from build123d import *

# Parameters (mm, degrees)
F0_R     = 2.8575
F1_DEPTH = 25.4


with BuildPart() as f1:
    # F0 (on Top) → F1 (new body)
    with BuildSketch(Plane.XY):
        with BuildLine():
            ThreePointArc((5.074602, 54.878098), (0, 60.192224), (-5.074602, 54.878098))
            ThreePointArc((-5.074602, 54.878098), (0, -55.112224), (5.074602, 54.878098))
        make_face()
        with BuildLine():
            ThreePointArc((43.232637, 12.702506), (44.60091, 6.416646), (45.060121, 0))
            ThreePointArc((45.060121, 0), (37.071988, -25.614102), (15.939817, -42.146611))
            ThreePointArc((15.939817, -42.146611), (13.779025, -42.901667), (11.582679, -43.546023))
            ThreePointArc((11.582679, -43.546023), (0, -45.060121), (-11.582679, -43.546023))
            ThreePointArc((-11.582679, -43.546023), (-13.779025, -42.901667), (-15.939817, -42.146611))
            ThreePointArc((-15.939817, -42.146611), (-40.341681, -20.073946), (-43.232637, 12.702506))
            ThreePointArc((-43.232637, 12.702506), (-40.292177, 20.173126), (-36.072623, 27.00334))
            ThreePointArc((-36.072623, 27.00334), (-30.371021, 33.286869), (-23.592574, 38.390168))
            ThreePointArc((-23.592574, 38.390168), (-17.875835, 41.362653), (-11.793582, 43.489378))
            ThreePointArc((-11.793582, 43.489378), (0, 45.060121), (11.793582, 43.489378))
            ThreePointArc((11.793582, 43.489378), (17.875835, 41.362653), (23.592574, 38.390168))
            ThreePointArc((23.592574, 38.390168), (30.371021, 33.286869), (36.072623, 27.00334))
            ThreePointArc((36.072623, 27.00334), (40.292177, 20.173126), (43.232637, 12.702506))
        make_face(mode=Mode.SUBTRACT)
        with Locations((0, 55.112224)):
            Circle(F0_R, mode=Mode.SUBTRACT)
        with BuildLine():
            Line((5.456394, 1.858352), (23.592574, 38.390168))
            ThreePointArc((23.592574, 38.390168), (17.875835, 41.362653), (11.793582, 43.489378))
            Line((11.793582, 43.489378), (0, 14.776533))
            Line((0, 14.776533), (-11.793582, 43.489378))
            ThreePointArc((-11.793582, 43.489378), (-17.875835, 41.362653), (-23.592574, 38.390168))
            Line((-23.592574, 38.390168), (-5.456394, 1.858352))
            Line((-5.456394, 1.858352), (0, 1.858352))
            Line((0, 1.858352), (5.456394, 1.858352))
        make_face()
        with BuildLine():
            Line((15.939817, -42.146611), (43.232637, 12.702506))
            ThreePointArc((43.232637, 12.702506), (40.292177, 20.173126), (36.072623, 27.00334))
            Line((36.072623, 27.00334), (13.962634, -21.160696))
            Line((13.962634, -21.160696), (5.882978, -1.074824))
            Line((5.882978, -1.074824), (0, -1.074824))
            Line((0, -1.074824), (-5.882978, -1.074824))
            Line((-5.882978, -1.074824), (-13.962634, -21.160696))
            Line((-13.962634, -21.160696), (-36.072623, 27.00334))
            ThreePointArc((-36.072623, 27.00334), (-40.292177, 20.173126), (-43.232637, 12.702506))
            Line((-43.232637, 12.702506), (-15.939817, -42.146611))
            ThreePointArc((-15.939817, -42.146611), (-13.779025, -42.901667), (-11.582679, -43.546023))
            Line((-11.582679, -43.546023), (0, -12.311705))
            Line((0, -12.311705), (11.582679, -43.546023))
            ThreePointArc((11.582679, -43.546023), (13.779025, -42.901667), (15.939817, -42.146611))
        make_face()
    extrude(amount=F1_DEPTH)


solid = f1.part
Design review of the part built by this model. Coordinates are the model's own, in mm. Coordinates: 2 decimals unless noted, no trailing zeros. Order: outer loops, then holes, each group sorted by start corner. A loop starts at its lowest first (then second) coordinate and runs counter-clockwise, first axis right, second up. Notation, with made-up numbers: (27, 20.25) -> (44, 20.25) arc R8 cw to (44, 33.25) -> close; hole circle Ø5 at (-27, 28.5). An arc over 180 degrees is marked (long way). One line per item, written item: value.
1) We need section C-C, the plane y = -9. Give the boundary of the cut face in (x, z), then the cut area to 3 significant figures.
Output values:
outline: (-54.37, 0) -> (-44.15, 0) -> (-44.15, 25.4) -> (-54.37, 25.4) -> close; (-32.43, 0) -> (-19.55, 0) -> (-19.55, 25.4) -> (-32.43, 25.4) -> close; (-9.07, 0) -> (9.07, 0) -> (9.07, 25.4) -> (-9.07, 25.4) -> close; (19.55, 0) -> (32.43, 0) -> (32.43, 25.4) -> (19.55, 25.4) -> close; (44.15, 0) -> (54.37, 0) -> (54.37, 25.4) -> (44.15, 25.4) -> close
area: 1,630 mm2
2) To check wall thickness, follow probe 1 along X at (y, z) = (27, 15); probe 2 along X at (y, z) = (-36, 7); probe 3 along X at (y, z) = (-14, 12.5). State the ranges of each line that lie inside material, in increasing order. Write a range as [from, to].
Output values:
probe 1: x = [-48.05, -36.07], [-17.94, -5.02], [5.02, 17.94], [36.07, 48.05]
probe 2: x = [-41.73, -27.1], [-19, -8.78], [8.78, 19], [27.1, 41.73]
probe 3: x = [-53.3, -42.83], [-29.95, -17.25], [-11.08, -0.63], [0.63, 11.08], [17.25, 29.95], [42.83, 53.3]
3) We need section B-B, the plane x = 21.5. Give the boundary of the cut face in (y, z).
Output values:
outline: (-50.75, 0) -> (-39.6, 0) -> (-39.6, 25.4) -> (-50.75, 25.4) -> close; (-30.97, 0) -> (-4.74, 0) -> (-4.74, 25.4) -> (-30.97, 25.4) -> close; (34.18, 0) -> (50.75, 0) -> (50.75, 25.4) -> (34.18, 25.4) -> close
4) We need section D-D, the plane z = 4.75. Give the boundary of the cut face in (x, y) (1 decimal), then the cut area to 3 significant figures.
Output values:
outline: (-5.1, 54.9) arc R55.1 ccw (long way) to (5.1, 54.9) arc R5.1 ccw (long way) to start; hole (-43.2, 12.7) arc R45.1 ccw to (-15.9, -42.1) -> close; hole (-36.1, 27) -> (-14, -21.2) -> (-5.9, -1.1) -> (5.9, -1.1) -> (14, -21.2) -> (36.1, 27) arc R45.1 ccw to (23.6, 38.4) -> (5.5, 1.9) -> (-5.5, 1.9) -> (-23.6, 38.4) arc R45.1 ccw to start; hole (-11.8, 43.5) -> (0, 14.8) -> (11.8, 43.5) arc R45.1 ccw to start; hole (-11.6, -43.5) arc R45.1 ccw to (11.6, -43.5) -> (0, -12.3) -> close; hole circle Ø5.7 at (0, 55.1); hole (15.9, -42.1) arc R45.1 ccw to (45.1, 0) arc R45.1 ccw to (43.2, 12.7) -> close
area: 6,150 mm2
5) We need section A-A, the plane y = 24. Give the boundary of the cut face in (x, z), then the cut area to 3 significant figures.
Output values:
outline: (-49.61, 0) -> (-34.69, 0) -> (-34.69, 25.4) -> (-49.61, 25.4) -> close; (-16.45, 0) -> (-3.79, 0) -> (-3.79, 25.4) -> (-16.45, 25.4) -> close; (3.79, 0) -> (16.45, 0) -> (16.45, 25.4) -> (3.79, 25.4) -> close; (34.69, 0) -> (49.61, 0) -> (49.61, 25.4) -> (34.69, 25.4) -> close
area: 1,400 mm2
6) Clearance check with flat-ended pins moving along their axes: P1, Ø12, axis at x = 0.5, z = 15, coming from the -Y side; P2, Ø12, axis at y = 8, z = 5.5, coming from the +X side; P3, Ø1.5, axis at y = 34.5, z = 10, coming from the +X side; P4, Ø2, axis at x = 28.5, z = 23, coming from the +Y side. State where each tip first meets the part, or that it passes through.
Output values:
P1: stops at y = -55.11
P2: stops at x = 55.08
P3: stops at x = 43.57
P4: stops at y = 47.76
7) Draft analysis for pull direction X (two halves, no side actions). For faces 1 (the face through (-2.352, -55.062, 12.522)), 2 (the face through (-30.459, 33.207, 12.522)), state which applies: +X half, -X half, draft (parallel to the pull), parting line (faces both ways), or undercut.
Output values:
face 1: parting line
face 2: undercut
